Read the model definition and answer for the solid it produces. Units are mm, in the model's axes. A direction names the side the tool comes from. Coordinates: 2 decimals unless noted, no trailing zeros. Order: outer loops, then holes, each group sorted by start corner. A loop starts at its lowest first (then second) coordinate and runs counter-clockwise, first axis right, second up.
from build123d import *

# Parameters (mm, degrees)
F0_W     = 82.946875
F0_H     = 25.908
F0_R     = 3.3734375
F0_R_2   = 9.779
F1_DEPTH = 6.35
F2_R     = 0.889
F3_DEPTH = 3.2164930276
F4_R     = 5.08
F5_SIZE  = 0.508


with BuildPart() as f1:
    # F0 (on Top) → F1 (new body)
    with BuildSketch(Plane.XY):
        Rectangle(F0_W, F0_H)
        with Locations((-31.75, 0)):
            Circle(F0_R, mode=Mode.SUBTRACT)
        Circle(F0_R_2, mode=Mode.SUBTRACT)
        with Locations((31.75, 0)):
            Circle(F0_R, mode=Mode.SUBTRACT)
    extrude(amount=F1_DEPTH)

    # F2 (on face) → F3 (cut, through all)
    with BuildSketch(Plane.XZ.offset(12.954)):
        with Locations((0, 3.175)):
            Circle(F2_R)
    extrude(amount=-F3_DEPTH, mode=Mode.SUBTRACT)

    # F4
    f4_edges = [f1.edges().sort_by_distance(p)[0] for p in [
        (-41.473438, -12.954, 3.175),
        (41.473438, -12.954, 3.175),
        (41.473438, 12.954, 3.175),
        (-41.473438, 12.954, 3.175),
    ]]
    fillet(f4_edges, radius=F4_R)

    # F5
    f5_edges = [f1.edges().sort_by_distance(p)[0] for p in [
        (-35.123438, 0, 6.35),
        (28.376562, 0, 6.35),
        (-35.123438, 0, 0),
        (28.376562, 0, 0),
    ]]
    chamfer(f5_edges, length=F5_SIZE)


solid = f1.part
Q1. Determine the mould class of faces 3 (the flat face through (-1, -12.954, 2)), 4 (the cylindrical face through (-2.12, -9.546, 3.131)), 5 (the flat face through (-1, 12.954, 3)) for opening direction Y: +Y half, -Y half, draft (parallel to the pull), parting line (faces both ways), or undercut.
Q2. Which of the six approach directions +Z, -Z, +X, -X, +Y, -Y give full straight-line access (tool end or side, diameter ignored) to faces 1 (the flat face through (-10, 0, 6.35)), 2 (the cylindrical face through (0.478, -11.369, 3.925))?
Q3. The part is cut by section B-B, the plane x = 31.75. Determine the outline of the cut face in (y, z), then the cut area to 3 significant figures.
Q4. Straight lines are drawn through the part: L1, parallel to Y at x = 31.75, z = 1.9; L2, parallel to X at y = 0.5, z = 4.25; L3, parallel to X at y = -1.75, z = 3. For each, find the intervals that lie inside material, in ascending order.
Q5. The part is cut by section C-C, the plane y = 5. Determine the outline of the cut face in (x, z).
Q6. Each of these flat-tipped pins is pushed along its axis until it touches: P1, Ø4, axis at x = 9, y = -1, coming from the +Z side; P2, Ø1.1, axis at x = 0, z = 3.175, coming from the -Y side; P3, Ø1, axis at y = 10, z = 3, coming from the -X side; P4, Ø15.5, axis at x = 0, y = 0, coming from the -Z side. Where does it stop, or does it pass through?
Q7. The part is cut by section A-A, the plane y = 0. Determine the outline of the cut face in (x, z), then the cut area to 3 significant figures.
Computed values:
1. face 3: -Y half
1. face 4: undercut
1. face 5: +Y half
2. face 1: +Z, +X, -X, +Y, -Y
2. face 2: -Y
3. outline: (-12.95, 0) - (-3.88, 0) - (-3.37, 0.51) - (-3.37, 5.84) - (-3.88, 6.35) - (-12.95, 6.35) - close; (3.37, 0.51) - (3.88, 0) - (12.95, 0) - (12.95, 6.35) - (3.88, 6.35) - (3.37, 5.84) - close
3. area: 121 mm2
4. L1: y = -12.95 to -3.37, 3.37 to 12.95
4. L2: x = -41.47 to -35.09, -28.41 to -9.77, 9.77 to 28.41, 35.09 to 41.47
4. L3: x = -41.47 to -34.63, -28.87 to -9.62, 9.62 to 28.87, 34.63 to 41.47
5. outline: (-41.47, 0) - (-8.4, 0) - (-8.4, 6.35) - (-41.47, 6.35) - close; (8.4, 0) - (41.47, 0) - (41.47, 6.35) - (8.4, 6.35) - close
6. P1: stops at z = 6.35
6. P2: stops at y = 9.76
6. P3: stops at x = -41.21
6. P4: passes through
7. outline: (-41.47, 0) - (-35.63, 0) - (-35.12, 0.51) - (-35.12, 5.84) - (-35.63, 6.35) - (-41.47, 6.35) - close; (-28.38, 0.51) - (-27.87, 0) - (-9.78, 0) - (-9.78, 6.35) - (-27.87, 6.35) - (-28.38, 5.84) - close; (9.78, 0) - (27.87, 0) - (28.38, 0.51) - (28.38, 5.84) - (27.87, 6.35) - (9.78, 6.35) - close; (35.12, 0.51) - (35.63, 0) - (41.47, 0) - (41.47, 6.35) - (35.63, 6.35) - (35.12, 5.84) - close
7. area: 316 mm2
